Drawing for the job (mm, zero at the part's lowest x, y, z). A direction names the side the tool comes from. Give positions to 0.01 mm unless a question says otherwise; leave off trailing zeros. Loops run counter-clockwise (first coordinate to the right, second up) from the corner with the lowest first, then second, coordinate; pieces in that order, holes last.
1) Band-saw the part on C-C on x = 79.5. List the corners of the cut face in (y, z), then the cut area to 3 significant figures.
2) Flat gauge pins, fed straight in: P1, Ø1.5, axis at x = 73.5, z = 43.5, coming from the +Y side; P2, Ø8, axis at x = 15.5, y = 64.5, coming from the -Z side; P3, Ø8, axis at x = 32, y = 79.5, coming from the -Z side; P4, Ø5, axis at x = 24.5, y = 40, coming from the +Z side. Where does each tip first touch, or does it go through?
3) Band-saw the part on B-B on y = 45. List the corners of the cut face in (x, z).
4) 3-axis set-ups, long thin cutter, end or side, ignore diameter. For the marked faces 1, 2 and 3: which of +Z, -Z, +X, -X, +Y, -Y reach the whole face in a straight line?
5) Wall check: line 1 (Z direction, x = 59, y = 98.5); line 2 (Y direction, x = 68.5, z = 53) (1 decimal); line 3 (Y direction, x = 26, z = 70) (1 decimal). Give the ranges that are in metal, low to high.
6) Band-saw the part on A-A on x = 39.5. List the corners of the cut face in (y, z).
7) Band-saw the part on D-D on z = 36.5. List the corners of the cut face in (x, y).
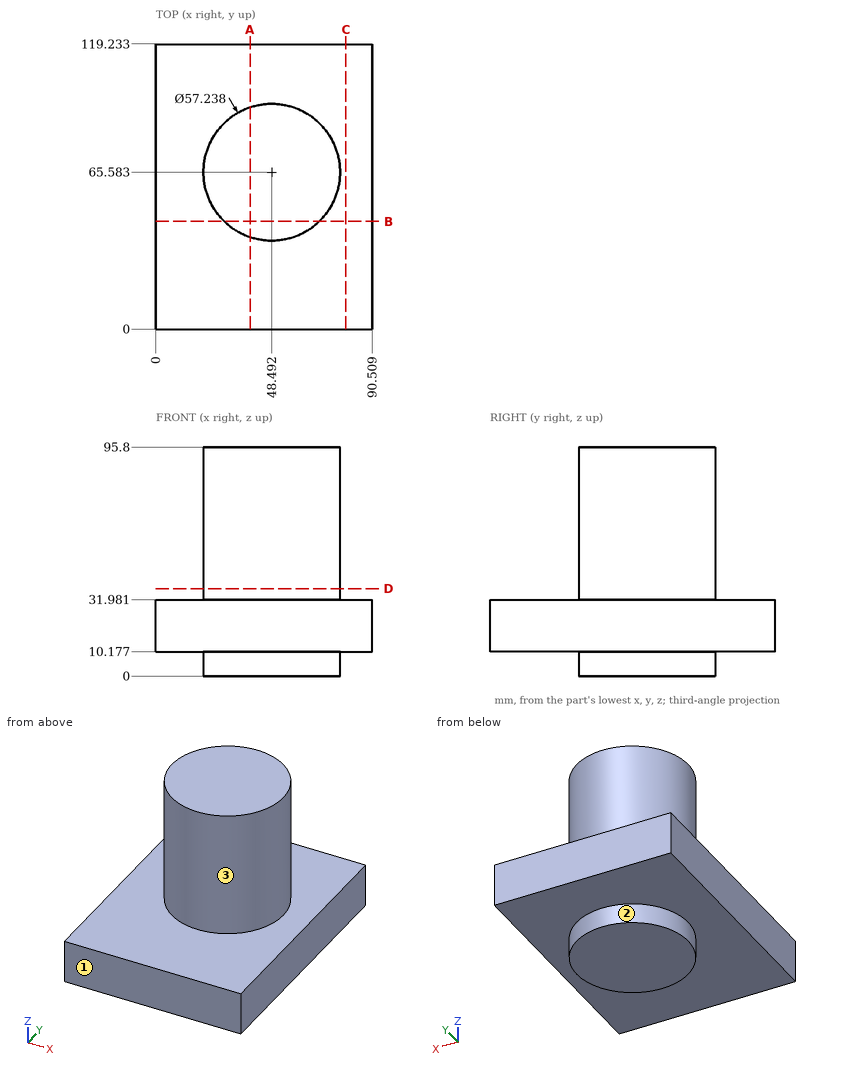
Findings below:
1. outline: (0, 10.18) - (119.23, 10.18) - (119.23, 31.98) - (0, 31.98) - close
1. area: 2,600 mm2
2. P1: stops at y = 80.77
2. P2: stops at z = 10.18
2. P3: stops at z = 0
2. P4: stops at z = 31.98
3. outline: (0, 10.18) - (28.61, 10.18) - (28.61, 0) - (68.38, 0) - (68.38, 10.18) - (90.51, 10.18) - (90.51, 31.98) - (68.38, 31.98) - (68.38, 95.8) - (28.61, 95.8) - (28.61, 31.98) - (0, 31.98) - close
4. face 1: +Z, -Z, +X, -X, -Y
4. face 2: -Z
4. face 3: +Z
5. line 1: z = 10.18 to 31.98
5. line 2: y = 45.1 to 86
5. line 3: y = 47.9 to 83.3
6. outline: (0, 10.18) - (38.41, 10.18) - (38.41, 0) - (92.75, 0) - (92.75, 10.18) - (119.23, 10.18) - (119.23, 31.98) - (92.75, 31.98) - (92.75, 95.8) - (38.41, 95.8) - (38.41, 31.98) - (0, 31.98) - close
7. outline: circle Ø57.24 at (48.49, 65.58)
